The listing builds one solid part. Answer for the finished solid, in the listing's coordinates (mm). A direction names the side the tool comes from. Give positions to 0.01 mm unless a question says otherwise; leave off trailing zeros. Loops run counter-clockwise (first coordinate to the right, second up) from the corner with the lowest first, then second, coordinate; pieces in that order, holes last. Notation, with made-up numbers: (29.25, -38.5) - (52.25, -38.5) arc R14 cw to (52.25, -29.5) - close; hole circle Ø3 at (-35, -8). An arc over 180 degrees is marked (long way). Write item = value, one per line. Start each with the question number.
1) Consider probe 1 along Z at (x, y) = (83.5, 3.75); probe 2 along Y at (x, z) = (94.5, -19.5); probe 3 along Z at (x, y) = (26, -0.75). Determine where each line is inside the solid, lowest interval first.
2) The part is cut by section A-A on x = 242.5. Write down the section's boundary in (y, z), plus the area to 3 significant figures.
3) Flat-ended cylindrical pins translate along their axes: P1, Ø4, axis at x = 272, z = -14.5, coming from the +Y side; P2, Ø12.5, axis at x = 109, y = 12.5, coming from the -Z side; P3, Ø0.9, axis at y = 12, z = 2, coming from the +X side. Find the tip coordinate at first contact, or state that the pin passes through.
4) The part is cut by section C-C on y = 3.25. Write down the section's boundary in (x, z).
5) Which of the six approach directions +Z, -Z, +X, -X, +Y, -Y give full straight-line access (tool end or side, diameter ignored) to faces 1 (the flat face through (170, 13, 0)), 2 (the flat face through (163, -3, -11))?
6) The part is cut by section B-B on z = -21.25. Write down the section's boundary in (x, y), plus the area to 3 significant figures.
from build123d import *

# Parameters (mm, degrees)
EXTRUDE_1_DEPTH     = 330
SKETCH_2_W          = 39
SKETCH_2_H          = 3
SKETCH_2_W_2        = 25
CUT_EXTRUDE_1_DEPTH = 29


with BuildPart() as part:
    # Эскиз1 → Вытянуть-Тонкостенный1 (new body)
    with BuildSketch(Plane(origin=(0, 0, 0), x_dir=(0, 0, -1), z_dir=(1, 0, 0))):
        Polygon((0, 25), (0, 0), (25, 0), (25, -3), (-3, -3), (-3, 25), align=None)
    extrude(amount=EXTRUDE_1_DEPTH)

    # Эскиз2 → Вырез-Вытянуть1 (cut, through all)
    with BuildSketch(Plane.XZ.offset(3)):
        with Locations((19.5, 1.5)):
            Rectangle(SKETCH_2_W, SKETCH_2_H)
        with Locations((317.5, 1.5)):
            Rectangle(SKETCH_2_W_2, SKETCH_2_H)
    extrude(amount=-CUT_EXTRUDE_1_DEPTH, mode=Mode.SUBTRACT)


solid = part.part
Answer below:
q1.probe_1 = 0 to 3
q1.probe_2 = -3 to 0
q1.probe_3 = -25 to 0
q2.outline = (-3, -25) - (0, -25) - (0, 0) - (25, 0) - (25, 3) - (-3, 3) - close
q2.area = 159 mm2
q3.P1 = 0
q3.P2 = 0
q3.P3 = 305
q4.outline = (39, 0) - (305, 0) - (305, 3) - (39, 3) - close
q5.face_1 = -Z, +X, -X, +Y
q5.face_2 = +Z, -Z, +X, -X, -Y
q6.outline = (0, -3) - (330, -3) - (330, 0) - (0, 0) - close
q6.area = 990 mm2
